Design review of the part shown in the three views and the two pictorial views. Dimensions are in mm from the part's minimum x, y and z. A direction names the side the tool comes from. Give positions to 0.01 mm unless a question says otherwise; leave off trailing zeros. Write each loop counter-clockwise with the first axis right and the second up, starting at its lowest first coordinate (ties: lowest second). Pieces come first, ordered by that corner, then holes. Notation, with made-up numbers: (44.5, 60) -> (57.5, 60) arc R24 ccw to (57.5, 88) -> close; hole circle Ø10 at (-36.75, 18.5). An arc over 180 degrees is marked (long way). Return JSON: item names as keys, results as strings. Group by question number.
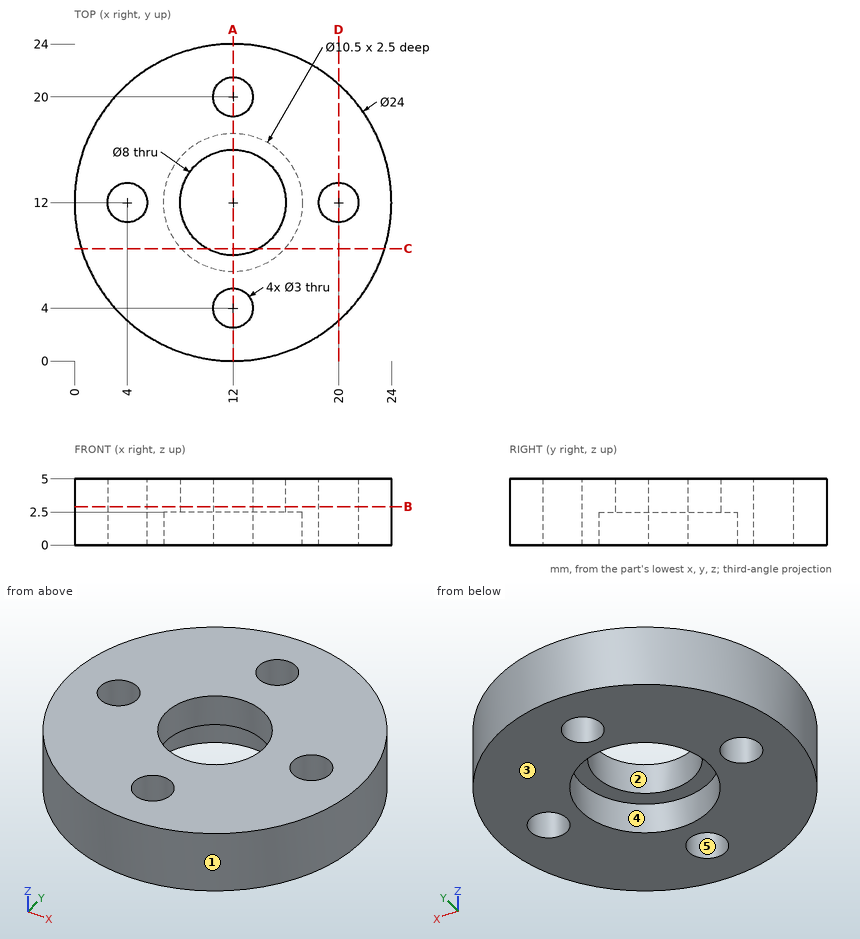
Q1. Take a section at B-B, the plane z = 2.9. Give the boundary of the cut face in (x, y), plus the area to 3 significant figures.
Q2. Tool access review of the marked faces 4 and 5: name each direction out of +Z, -Z, +X, -X, +Y, -Y from which nothing blocks a thin tool from reaching the whole face with its end or side.
Q3. For L1, parallel to X at y = 13.25, z = 0.5; L2, parallel to Y at x = 11.75, z = 4; L3, parallel to X at y = 4.5, z = 1, list the stretches that pass through material, from the lowest coordinate up. Write a range as from..to.
Q4. Insertion check: pin 1 (1.5 mm diameter, centred on x = 5, z = 0.5, fed in from -Y); pin 2 (1.5 mm diameter, centred on y = 5.5, z = 4, fed in from +X); pin 3 (5 mm diameter, centred on x = 10.5, y = 13, fed in from -Z). Each pin has a flat end and moves straight along its axis. Give the tip position at first contact, or say it passes through.
Q5. Take a section at D-D, the plane x = 20. Give the boundary of the cut face in (y, z), plus the area to 3 significant figures.
Q6. Take a section at A-A, the plane x = 12. Give the boundary of the cut face in (y, z).
Q7. Take a section at C-C, the plane y = 8.5. Give the boundary of the cut face in (x, z).
Q8. Mouldability with a two-part tool opening along Y and no side actions: class the marked faces 1, 2 and 3 as +Y half, -Y half, draft (parallel to the pull), parting line (faces both ways), or undercut.
Final values:
{
 "1": {"outline": "circle Ø24 at (12, 12); hole circle Ø3 at (4, 12); hole circle Ø8 at (12, 12); hole circle Ø3 at (12, 4); hole circle Ø3 at (12, 20); hole circle Ø3 at (20, 12)", "area": "374 mm²"},
 "2": {"face 4": "-Z", "face 5": "+Z, -Z"},
 "3": {"L1": "x = 0.07..3.17, 4.83..6.9, 17.1..19.17, 20.83..23.93", "L2": "y = 0..2.52, 5.48..8.01, 15.99..18.52, 21.48..24", "L3": "x = 2.63..10.59, 13.41..21.37"},
 "4": {"pin 1": "stops at y = 1.76", "pin 2": "stops at x = 22.53", "pin 3": "stops at z = 2.5"},
 "5": {"outline": "(3.06, 0) -> (10.5, 0) -> (10.5, 5) -> (3.06, 5) -> close; (13.5, 0) -> (20.94, 0) -> (20.94, 5) -> (13.5, 5) -> close", "area": "74.4 mm²"},
 "6": {"outline": "(0, 0) -> (2.5, 0) -> (2.5, 5) -> (0, 5) -> close; (5.5, 0) -> (6.75, 0) -> (6.75, 2.5) -> (8, 2.5) -> (8, 5) -> (5.5, 5) -> close; (16, 2.5) -> (17.25, 2.5) -> (17.25, 0) -> (18.5, 0) -> (18.5, 5) -> (16, 5) -> close; (21.5, 0) -> (24, 0) -> (24, 5) -> (21.5, 5) -> close"},
 "7": {"outline": "(0.52, 0) -> (8.09, 0) -> (8.09, 2.5) -> (10.06, 2.5) -> (10.06, 5) -> (0.52, 5) -> close; (13.94, 2.5) -> (15.91, 2.5) -> (15.91, 0) -> (23.48, 0) -> (23.48, 5) -> (13.94, 5) -> close"},
 "8": {"face 1": "parting line", "face 2": "undercut", "face 3": "draft"}
}
